```python
from build123d import *


with BuildPart() as part:
    # Sketch1 → Revolve1 (revolve)
    with BuildSketch(Plane.XY, mode=Mode.PRIVATE) as revolve1_sk:
        Polygon((2.75, 6.35), (1.2, 6.35), (1.2, 9.6), (0.75, 10.05), (0.75, 10.6), (1.2, 10.6), (1.2, 10.9), (0.75, 11.35), (0.75, 11.9), (1.2, 11.9), (1.2, 12.2), (0.4, 13), (0, 13), (0, 0), (2.75, 0), align=None)
    revolve(revolve1_sk.sketch.rotate(Axis((0, 0, 0), (0, -1, 0)), 180), axis=Axis((0, 0, 0), (0, -1, 0)))  # turned: the seam where the file's is


solid = part.part
```
Work out the finished part from the listing and answer in its coordinate system (mm). A direction names the side the tool comes from. Give positions to 0.01 mm unless a question says otherwise; leave off trailing zeros. Order: outer loops, then holes, each group sorted by start corner. A loop starts at its lowest first (then second) coordinate and runs counter-clockwise, first axis right, second up. Notation, with made-up numbers: M 46,1.25 L 56,1.25 A16 ccw 56,22.25 Z; hole C 52,-33.5 d10. An arc over 180 degrees is marked long. Return JSON: item names as keys, results as strings.
1) A tool of negligible diameter and unlimited length cuts with its end or side. For faces 4 (the flat face through (0, 0, 0)), 5 (the cylindrical face through (-0.65, 8, -1.01)), 6 (the flat face through (0, 10.6, 1)), from which of +Z, -Z, +X, -X, +Y, -Y can it reach the whole face along a straight path? Write none if from no direction.
Resolved:
{"face 4": "+Z, -Z, +X, -X, -Y", "face 5": "+Y", "face 6": "none"}
2) Straight lines are drawn through the part: line 1 along Y through (x, z) = (1.05, 0.45); line 2 along Y through (x, z) = (-1.95, 1.5); line 3 along Z through (x, y) = (-0.05, 8). For each, find the intervals that lie inside material, in ascending order. Write a range as [from, to].
Resolved:
{"line 1": "[0, 9.66], [10.6, 10.96], [11.9, 12.26]", "line 2": "[0, 6.35]", "line 3": "[-1.2, 1.2]"}
3) Section D-D, the plane z = 0.9 is taken. Give the number of separate pieces and of enclosed holes in the cut face, plus the area to 3 significant figures.
Resolved:
{"separate pieces": "3", "enclosed holes": "0", "area": "40.0 mm^2"}
4) Each of these flat-tipped pins is pushed along its axis until it touches: pin 1 (3 mm diameter, centred on x = -0.5, y = 11.5, fed in from -Z); pin 2 (2 mm diameter, centred on x = 1.5, y = 10.5, fed in from -Z). Where does it stop, or does it pass through?
Resolved:
{"pin 1": "z = -1.2", "pin 2": "z = -1.09"}
5) Section C-C, the plane y = 8.75 is taken. Write down the section's boundary in (x, z).
Resolved:
{"outline": "C 0,0 d2.4"}
6) For a pull along Y with two mould halves and no side action, classify faces 1 (the flat face through (0, 11.9, 1)), 2 (the cylindrical face through (0.596, 3.219, 2.685)), 3 (the flat face through (-1, 6.35, 1)) as +Y half, -Y half, draft (parallel to the pull), parting line (faces both ways), or undercut.
Resolved:
{"face 1": "undercut", "face 2": "draft", "face 3": "+Y half"}
7) Section A-A, the plane x = 0 is taken. Write down the section's boundary in (y, z).
Resolved:
{"outline": "M 0,-2.75 L 6.35,-2.75 L 6.35,-1.2 L 9.6,-1.2 L 10.05,-0.75 L 10.6,-0.75 L 10.6,-1.2 L 10.9,-1.2 L 11.35,-0.75 L 11.9,-0.75 L 11.9,-1.2 L 12.2,-1.2 L 13,-0.4 L 13,0.4 L 12.2,1.2 L 11.9,1.2 L 11.9,0.75 L 11.35,0.75 L 10.9,1.2 L 10.6,1.2 L 10.6,0.75 L 10.05,0.75 L 9.6,1.2 L 6.35,1.2 L 6.35,2.75 L 0,2.75 Z"}
8) Section B-B, the plane z = 0 is taken. Write down the section's boundary in (x, y).
Resolved:
{"outline": "M -2.75,0 L 2.75,0 L 2.75,6.35 L 1.2,6.35 L 1.2,9.6 L 0.75,10.05 L 0.75,10.6 L 1.2,10.6 L 1.2,10.9 L 0.75,11.35 L 0.75,11.9 L 1.2,11.9 L 1.2,12.2 L 0.4,13 L -0.4,13 L -1.2,12.2 L -1.2,11.9 L -0.75,11.9 L -0.75,11.35 L -1.2,10.9 L -1.2,10.6 L -0.75,10.6 L -0.75,10.05 L -1.2,9.6 L -1.2,6.35 L -2.75,6.35 Z"}
